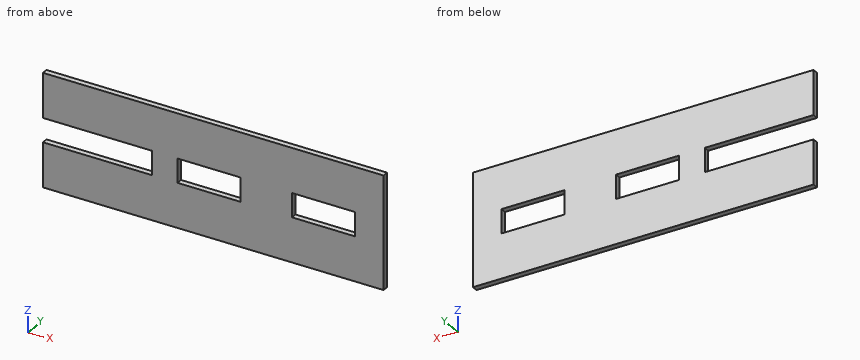
from build123d import *

# Parameters (mm, degrees)
SKETCH1_W           = 119
SKETCH1_H           = 40
BOSS_EXTRUDE1_DEPTH = 2
SKETCH2_W           = 38
SKETCH2_H           = 8.5
CUT_EXTRUDE1_DEPTH  = 3
SKETCH3_W           = 22
SKETCH3_H           = 8.5
CUT_EXTRUDE2_DEPTH  = 3


with BuildPart() as part:
    # Sketch1 → Boss-Extrude1 (new body)
    with BuildSketch(Plane(origin=(0, 0, 0), x_dir=(1, 0, 0), z_dir=(0, 1, 0))):
        with Locations((59.5, -20)):
            Rectangle(SKETCH1_W, SKETCH1_H)
    extrude(amount=BOSS_EXTRUDE1_DEPTH)

    # Sketch2 → Cut-Extrude1 (cut, through all)
    with BuildSketch(Plane(origin=(0, 2, 0), x_dir=(1, 0, 0), z_dir=(0, 1, 0))):
        with Locations((19, -20)):
            Rectangle(SKETCH2_W, SKETCH2_H)
    extrude(amount=-CUT_EXTRUDE1_DEPTH, mode=Mode.SUBTRACT)

    # Sketch3 → Cut-Extrude2 (cut, through all)
    with BuildSketch(Plane(origin=(0, 2, 0), x_dir=(1, 0, 0), z_dir=(0, 1, 0))):
        with Locations((58, -20)):
            Rectangle(SKETCH3_W, SKETCH3_H)
        with Locations((98, -20)):
            Rectangle(SKETCH3_W, SKETCH3_H)
    extrude(amount=-CUT_EXTRUDE2_DEPTH, mode=Mode.SUBTRACT)


solid = part.part
CAD build for the part. Positions are in the model's coordinates, mm. Coordinates: 2 decimals unless noted, no trailing zeros. Write each loop counter-clockwise with the first axis right and the second up, starting at its lowest first coordinate (ties: lowest second). Pieces come first, ordered by that corner, then holes. Notation, with made-up numbers: (8.25, -18) - (23.25, -18) arc R22 cw to (23.25, 10) - close; hole circle Ø4 at (1.5, 62). An arc over 180 degrees is marked (long way). Use a Markdown table: item, result. Add a question column.
Item 1: Drill centre lines: L1, parallel to Z at x = 62, y = 0.95; L2, parallel to X at y = 0.7, z = 16. Where is each one in solid material? Low to high. Write a range as from..to.
Item 2: Flat gauge pin, fed straight in: pin 1 (0.6 mm diameter, centred on y = 0.5, z = 22, fed in from -X). Where does the tip first touch, or does it go through?
Item 3: Band-saw the part on A-A, the plane y = 1.65. Give the cut face in (x, z).
Item 4: Band-saw the part on B-B, the plane x = 62. Give the cut face in (y, z).
Item 5: Band-saw the part on C-C, the plane z = 22. Give the cut face in (x, y), and give its area (3 significant figures).
Numbers:
| question | item | result |
|---|---|---|
| 1 | L1 | 0..15.75, 24.25..40 |
| 1 | L2 | 38..47, 69..87, 109..119 |
| 2 | pin 1 | x = 38 |
| 3 | outline | (0, 0) - (119, 0) - (119, 40) - (0, 40) - (0, 24.25) - (38, 24.25) - (38, 15.75) - (0, 15.75) - close; hole (47, 15.75) - (69, 15.75) - (69, 24.25) - (47, 24.25) - close; hole (87, 15.75) - (109, 15.75) - (109, 24.25) - (87, 24.25) - close |
| 4 | outline | (0, 0) - (2, 0) - (2, 15.75) - (0, 15.75) - close; (0, 24.25) - (2, 24.25) - (2, 40) - (0, 40) - close |
| 5 | outline | (38, 0) - (47, 0) - (47, 2) - (38, 2) - close; (69, 0) - (87, 0) - (87, 2) - (69, 2) - close; (109, 0) - (119, 0) - (119, 2) - (109, 2) - close |
| 5 | area | 74.0 mm2 |
